```python
from build123d import *

# Parameters (mm, degrees)
SKETCH_2_W          = 13.4
SKETCH_2_H          = 12
SKETCH_2_R          = 3.5
EXTRUDE_2_DEPTH     = 15
SKETCH_3_W          = 10
SKETCH_3_H          = 11
CUT_EXTRUDE_1_DEPTH = 11


with BuildPart() as part:
    # 草图2 → 凸台-拉伸2 (new body)
    with BuildSketch(Plane(origin=(0, 0, 0), x_dir=(1, 0, 0), z_dir=(0, 1, 0))):
        with Locations((6.7, -6)):
            Rectangle(SKETCH_2_W, SKETCH_2_H)
        with Locations(Location((8.395740059, -6, 0), (0, 0, 270))):
            Circle(SKETCH_2_R, mode=Mode.SUBTRACT)
    extrude(amount=EXTRUDE_2_DEPTH)

    # 草图3 → 切除-拉伸1 (cut)
    with BuildSketch(Plane.XZ):
        with Locations((8.4, 6)):
            Rectangle(SKETCH_3_W, SKETCH_3_H)
    extrude(amount=-CUT_EXTRUDE_1_DEPTH, mode=Mode.SUBTRACT)


solid = part.part
```
Can you work these out from the model? Positions are in its coordinate system, mm. A direction names the side the tool comes from. Coordinates: 2 decimals unless noted, no trailing zeros. Loops run counter-clockwise (first coordinate to the right, second up) from the corner with the lowest first, then second, coordinate; pieces in that order, holes last.
1) Imagine slicing it at D-D on z = 3. List the corners of the cut face in (x, y) for me.
2) Imagine slicing it at A-A on z = 6. List the corners of the cut face in (x, y) for me.
3) Imagine slicing it at B-B on x = 9.5. List the corners of the cut face in (y, z) for me, plus the area to 3 significant figures.
4) For pin 1 (1.5 mm diameter, centred on y = 7, z = 8.5, fed in from +X); pin 2 (6.5 mm diameter, centred on x = 8.4, z = 6, fed in from +Y), each with a flat end and sliding along its axis, tell me the tip position at first contact or that it passes through.
5) Imagine slicing it at C-C on y = 4.25. List the corners of the cut face in (x, z) for me.
6) Which directions (+Z, -Z, +X, -X, +Y, -Y) give clear straight access to the entire face, cutting with the end or side of a thin tool? Please do faces 5 (the flat face through (3.4, 5, 6)), 6 (the flat face through (4, 15, 6)).
7) I need wall thicknesses on probe 1 along Z at (x, y) = (12.75, 1.75); probe 2 along X at (y, z) = (14.05, 6); probe 3 along X at (y, z) = (8.5, 10.75). Which ranges of each line are inside material? Lowest first, please.
8) Thinking about a two-plate mould opening in Z: for faces 1 (the flat face through (7, 7, 0)), 2 (the flat face through (8, 5, 11.5)), 3 (the flat face through (12, 11, 7)), 4 (the flat face through (13.4, 11.4, 6)), which applies, pulls with the +Z half, pulls with the -Z half, needs draft (parallel to the pull), parting line crosses it, or undercut?
Completed:
1. outline: (0, 0) - (3.4, 0) - (3.4, 11) - (6.59, 11) - (6.59, 15) - (0, 15) - close; (10.2, 11) - (13.4, 11) - (13.4, 15) - (10.2, 15) - close
2. outline: (0, 0) - (3.4, 0) - (3.4, 11) - (4.9, 11) - (4.9, 15) - (0, 15) - close; (11.9, 11) - (13.4, 11) - (13.4, 15) - (11.9, 15) - close
3. outline: (0, 0) - (15, 0) - (15, 2.68) - (11, 2.68) - (11, 0.5) - (0, 0.5) - close; (0, 11.5) - (11, 11.5) - (11, 9.32) - (15, 9.32) - (15, 12) - (0, 12) - close
3. area: 32.4 mm2
4. pin 1: stops at x = 3.4
4. pin 2: passes through
5. outline: (0, 0) - (13.4, 0) - (13.4, 0.5) - (3.4, 0.5) - (3.4, 11.5) - (13.4, 11.5) - (13.4, 12) - (0, 12) - close
6. face 5: +X, -Y
6. face 6: +Z, -Z, +X, -X, +Y
7. probe 1: z = 0 to 0.5, 11.5 to 12
7. probe 2: x = 0 to 4.9, 11.9 to 13.4
7. probe 3: x = 0 to 3.4
8. face 1: pulls with the -Z half
8. face 2: undercut
8. face 3: undercut
8. face 4: needs draft
